Part model, mm, in its own coordinate system. Coordinates: 2 decimals unless noted, no trailing zeros. Order: outer loops, then holes, each group sorted by start corner. A loop starts at its lowest first (then second) coordinate and runs counter-clockwise, first axis right, second up. Notation, with made-up numbers: M 36.5,65 L 84.5,65 A35 ccw 84.5,103 Z; hole C -39,26 d1. An arc over 180 degrees is marked long. Answer in a Markdown table with one row per item. Add a question column.
from build123d import *

# Parameters (mm, degrees)
SKETCH1_R                                 = 19.05
BILLET_DEPTH                              = 3.81
SKETCH2_R                                 = 0.6477
FIRST_LOX_HOLE_DEPTH                      = 28.208842313
BRAISING_CHAMFER_SIZE                     = 0.254
LOX_HOLE_PATTERN_COUNT                    = 7
LOX_HOLE_PATTERN_PITCH                    = 2.9972
LOX_HOLE_PATTERN_COUNT_DIR2               = 7
LOX_HOLE_PATTERN_PITCH_DIR2               = 2.9972
BRAISING_CHAMFER_OF_LOX_HOLE_PATTERN_SIZE = 0.254


with BuildPart() as part:
    # Sketch1 → Billet (new body)
    with BuildSketch(Plane(origin=(0, 0, 0), x_dir=(1, 0, 0), z_dir=(0, 1, 0))):
        with Locations(Location((0, 0, 0), (0, 0, 270))):
            Circle(SKETCH1_R)
    extrude(amount=-BILLET_DEPTH)

    # Sketch2 → First Lox Hole (cut, symmetric)
    with BuildSketch(Plane(origin=(0, 0, 0), x_dir=(1, 0, 0), z_dir=(0, 1, 0))):
        with Locations(Location((8.9916, 8.9916, 0), (0, 0, 270))):
            Circle(SKETCH2_R)
    first_lox_hole = extrude(amount=FIRST_LOX_HOLE_DEPTH, both=True, mode=Mode.SUBTRACT)

    # Braising Chamfer
    braising_chamfer_edges = [part.edges().sort_by_distance(p)[0] for p in [
        (8.9916, -3.81, -9.6393),
    ]]
    chamfer(braising_chamfer_edges, length=BRAISING_CHAMFER_SIZE)

    # Lox Hole Pattern: First Lox Hole 7 × 7, 5 skipped
    with Locations(*[(-i * LOX_HOLE_PATTERN_PITCH, 0, j * LOX_HOLE_PATTERN_PITCH_DIR2) for i in range(LOX_HOLE_PATTERN_COUNT) for j in range(LOX_HOLE_PATTERN_COUNT_DIR2) if (i, j) not in ((0, 0), (2, 2), (2, 4), (3, 3), (4, 2), (4, 4))]):
        add(first_lox_hole, mode=Mode.SUBTRACT)

    # Braising Chamfer of Lox Hole Pattern
    braising_chamfer_of_lox_hole_pattern_edges = [part.edges().sort_by_distance(p)[0] for p in [
        (8.9916, -3.81, -6.6421),
        (8.9916, -3.81, -3.6449),
        (8.9916, -3.81, -0.6477),
        (8.9916, -3.81, 2.3495),
        (8.9916, -3.81, 5.3467),
        (8.9916, -3.81, 8.3439),
        (5.9944, -3.81, -9.6393),
        (5.9944, -3.81, -6.6421),
        (5.9944, -3.81, -3.6449),
        (5.9944, -3.81, -0.6477),
        (5.9944, -3.81, 2.3495),
        (5.9944, -3.81, 5.3467),
        (5.9944, -3.81, 8.3439),
        (2.9972, -3.81, -9.6393),
        (2.9972, -3.81, -6.6421),
        (2.9972, -3.81, -0.6477),
        (2.9972, -3.81, 5.3467),
        (2.9972, -3.81, 8.3439),
        (0, -3.81, -9.6393),
        (0, -3.81, -6.6421),
        (0, -3.81, -3.6449),
        (0, -3.81, 2.3495),
        (0, -3.81, 5.3467),
        (0, -3.81, 8.3439),
        (-2.9972, -3.81, -9.6393),
        (-2.9972, -3.81, -6.6421),
        (-2.9972, -3.81, -0.6477),
        (-2.9972, -3.81, 5.3467),
        (-2.9972, -3.81, 8.3439),
        (-5.9944, -3.81, -9.6393),
        (-5.9944, -3.81, -6.6421),
        (-5.9944, -3.81, -3.6449),
        (-5.9944, -3.81, -0.6477),
        (-5.9944, -3.81, 2.3495),
        (-5.9944, -3.81, 5.3467),
        (-5.9944, -3.81, 8.3439),
        (-8.9916, -3.81, -9.6393),
        (-8.9916, -3.81, -6.6421),
        (-8.9916, -3.81, -3.6449),
        (-8.9916, -3.81, -0.6477),
        (-8.9916, -3.81, 2.3495),
        (-8.9916, -3.81, 5.3467),
        (-8.9916, -3.81, 8.3439),
    ]]
    chamfer(braising_chamfer_of_lox_hole_pattern_edges, length=BRAISING_CHAMFER_OF_LOX_HOLE_PATTERN_SIZE)


solid = part.part
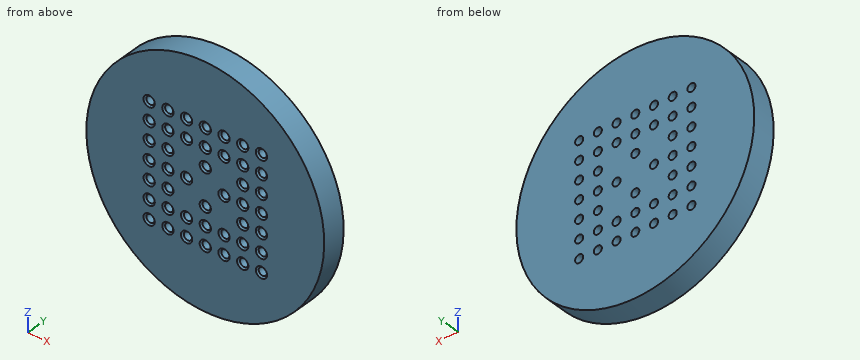
(1) Slice it at A-A (x = 0). State how many separate pieces and enclosed holes the cut face has, and give its area (3 significant figures).
(2) Drop flat-ended pins along their axis: P1, Ø1.7, axis at x = -3, z = 8.99, coming from the -Y side; P2, Ø1.2, axis at x = -5.99, z = 3, coming from the -Y side; P3, Ø1.5, axis at x = -14, y = -2, coming from the -Z side. Give the stop position or say it passes through.
(3) Wall check: line 1 (X direction, y = -1.6, z = -2.5); line 2 (Z direction, x = 3, y = -0.55); line 3 (X direction, y = -1.85, z = 11). Give the ranges that are in metal, low to high.
(4) Slice it at D-D (z = 17). List the corners of the cut face in (x, y).
Computed:
| question | item | result |
|---|---|---|
| 1 | separate pieces | 7 |
| 1 | enclosed holes | 0 |
| 1 | area | 115 mm^2 |
| 2 | P1 | stops at y = -3.76 |
| 2 | P2 | passes through |
| 2 | P3 | stops at z = -13.69 |
| 3 | line 1 | x = -18.89 to -9.41, -8.58 to -6.41, -5.58 to -0.42, 0.42 to 5.58, 6.41 to 8.58, 9.41 to 18.89 |
| 3 | line 2 | z = -18.81 to -9.64, -8.34 to -6.64, -5.35 to -0.65, 0.65 to 5.35, 6.64 to 8.34, 9.64 to 18.81 |
| 3 | line 3 | x = -15.55 to 15.55 |
| 4 | outline | M -8.6,-3.81 L 8.6,-3.81 L 8.6,0 L -8.6,0 Z |
